from build123d import *

# Parameters (mm, degrees)
SKETCH_1_R      = 1.5
SKETCH_1_R_2    = 8.5
EXTRUDE_1_DEPTH = 4


with BuildPart() as part:
    # 草图1 → 凸台-拉伸1 (new body)
    with BuildSketch(Plane(origin=(0, 0, 0), x_dir=(0, 0, -1), z_dir=(1, 0, 0))):
        with BuildLine():
            Line((-10, 26), (-10, -21))
            ThreePointArc((-10, -21), (0, -31), (10, -21))
            Line((10, -21), (10, 26))
            Line((10, 26), (-10, 26))
        make_face()
        with Locations((0, 22.5)):
            Circle(SKETCH_1_R, mode=Mode.SUBTRACT)
        with Locations((0, -21)):
            Circle(SKETCH_1_R_2, mode=Mode.SUBTRACT)
        with Locations((0, -2.5)):
            Circle(SKETCH_1_R, mode=Mode.SUBTRACT)
    extrude(amount=EXTRUDE_1_DEPTH)


solid = part.part
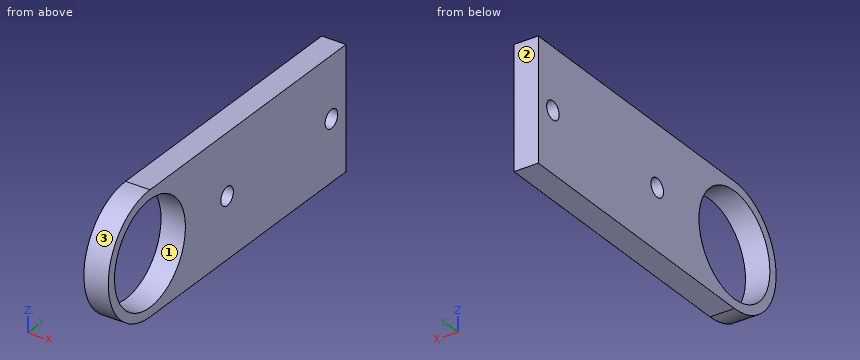
Input: part model. Units: mm. Frame: model coordinates. Face numbers are marked on the shaded views. Round coordinates to 2 decimals unless told otherwise and drop trailing zeros. Order: outer loops, then holes, each group sorted by start corner. A loop starts at its lowest first (then second) coordinate and runs counter-clockwise, first axis right, second up. Notation, with made-up numbers: (31.5, -6.75) - (90.5, -6.75) arc R21 ccw to (90.5, 14.25) - close; hole circle Ø1 at (35, -19.5). An arc over 180 degrees is marked (long way). Answer as a JSON object with one key per item and string values. Group by question number.
(1) Cut plane A-A (z = 0). Return loops of the section in (x, y), then the cut area to 3 significant figures.
(2) Cut plane B-B (y = 22.5). Return loops of the section in (x, z), then the cut area to 3 significant figures.
(3) Cut plane C-C (x = 2.6). Return loops of the section in (y, z), then the cut area to 3 significant figures.
(4) Material intervals for probe 1 along Y at (x, z) = (3.15, 0); probe 2 along Z at (x, y) = (2.9, -26); probe 3 along Y at (x, z) = (2.4, -1), sorted ascending. Write a range as from..to.
(5) Pin query (flat end, axial travel): P1, Ø5, axis at y = -22.5, z = 3.5, coming from the +X side. Return the tip coordinate at first contact, or that it passes through.
(6) Cut plane D-D (z = -3.5). Return loops of the section in (x, y), then the cut area to 3 significant figures.
(7) Draft query along Z for the marked faces 1, 2 and 3. Return one class per face: released by +Z, released by -Z, zero draft, split by the parting line, or undercut.
Here are the results:
{
 "1": {"outline": "(0, -31) - (4, -31) - (4, -29.5) - (0, -29.5) - close; (0, -12.5) - (4, -12.5) - (4, -4) - (0, -4) - close; (0, -1) - (4, -1) - (4, 21) - (0, 21) - close; (0, 24) - (4, 24) - (4, 26) - (0, 26) - close", "area": "136 mm^2"},
 "2": {"outline": "(0, -10) - (4, -10) - (4, -1.5) - (0, -1.5) - close; (0, 1.5) - (4, 1.5) - (4, 10) - (0, 10) - close", "area": "68.0 mm^2"},
 "3": {"outline": "(-21, -10) - (26, -10) - (26, 10) - (-21, 10) arc R10 ccw to start; hole circle Ø17 at (-21, 0); hole circle Ø3 at (-2.5, 0); hole circle Ø3 at (22.5, 0)", "area": "856 mm^2"},
 "4": {"probe 1": "y = -31..-29.5, -12.5..-4, -1..21, 24..26", "probe 2": "z = -8.66..-6.87, 6.87..8.66", "probe 3": "y = -30.95..-29.44, -12.56..-3.62, -1.38..21.38, 23.62..26"},
 "5": {"P1": "passes through"},
 "6": {"outline": "(0, -30.37) - (4, -30.37) - (4, -28.75) - (0, -28.75) - close; (0, -13.25) - (4, -13.25) - (4, 26) - (0, 26) - close", "area": "164 mm^2"},
 "7": {"face 1": "undercut", "face 2": "zero draft", "face 3": "split by the parting line"}
}
